```python
from build123d import *

# Parameters (mm, degrees)
SKETCH1_W           = 13.5
SKETCH1_H           = 13.5
BOSS_EXTRUDE1_DEPTH = 5
SKETCH3_W           = 13.5
SKETCH3_H           = 13.5
BOSS_EXTRUDE2_DEPTH = 2
CHAMFER1_SIZE       = 2.5
FILLET2_R           = 0.5
FILLET1_R           = 0.5
CUT_EXTRUDE1_REACH  = 4
SKETCH4_R           = 2.9
CHAMFER2_SIZE       = 0.2


with BuildPart() as part:
    # Sketch1 → Boss-Extrude1 (new body)
    with BuildSketch(Plane(origin=(0, 0, 0), x_dir=(1, 0, 0), z_dir=(0, 1, 0))):
        Rectangle(SKETCH1_W, SKETCH1_H)
        Polygon((0, -5.715767665), (4.95, -2.857883832), (4.95, 2.857883832), (0, 5.715767665), (-4.95, 2.857883832), (-4.95, -2.857883832), align=None, mode=Mode.SUBTRACT)
    extrude(amount=BOSS_EXTRUDE1_DEPTH)

    # Sketch3 → Boss-Extrude2 (add)
    with BuildSketch(Plane(origin=(0, 5, 0), x_dir=(1, 0, 0), z_dir=(0, 1, 0))):
        Rectangle(SKETCH3_W, SKETCH3_H)
    extrude(amount=BOSS_EXTRUDE2_DEPTH)

    # Chamfer1
    chamfer1_edges = [part.edges().sort_by_distance(p)[0] for p in [
        (-6.75, 7, 0),
        (6.75, 7, 0),
    ]]
    chamfer(chamfer1_edges, length=CHAMFER1_SIZE)

    # Fillet2
    fillet2_edges = [part.edges().sort_by_distance(p)[0] for p in [
        (-4.95, 2.5, 2.857883832),
        (0, 2.5, 5.715767665),
        (4.95, 2.5, 2.857883832),
        (4.95, 2.5, -2.857883832),
        (0, 2.5, -5.715767665),
        (-4.95, 2.5, -2.857883832),
    ]]
    fillet(fillet2_edges, radius=FILLET2_R)

    # Fillet1
    fillet1_edges = [part.edges().sort_by_distance(p)[0] for p in [
        (0, 7, 6.75),
        (0, 7, -6.75),
        (-4.25, 7, 0),
        (4.25, 7, 0),
        (-6.75, 2.25, -6.75),
        (6.75, 2.25, -6.75),
        (-5.5, 5.75, -6.75),
        (5.5, 5.75, -6.75),
        (6.75, 2.25, 6.75),
        (6.75, 4.5, 0),
        (-6.75, 2.25, 6.75),
        (-5.5, 5.75, 6.75),
        (5.5, 5.75, 6.75),
        (-6.75, 4.5, 0),
    ]]
    fillet(fillet1_edges, radius=FILLET1_R)

    # Sketch4 → Cut-Extrude1 (cut, up to next)
    with BuildSketch(Plane.XZ.offset(-5), mode=Mode.PRIVATE) as cut_extrude1_sk1:
        Circle(SKETCH4_R)
    cut_extrude1_tool1 = extrude(cut_extrude1_sk1.sketch, amount=-CUT_EXTRUDE1_REACH, mode=Mode.PRIVATE) & part.part
    add(cut_extrude1_tool1.solids().sort_by_distance((0, 5, 0))[0], mode=Mode.SUBTRACT)

    # Chamfer2
    chamfer2_edges = [part.edges().sort_by_distance(p)[0] for p in [
        (-2.9, 5, 0),
    ]]
    chamfer(chamfer2_edges, length=CHAMFER2_SIZE)


solid = part.part
```
Could you check a few things on this model? Use its own coordinates, in mm. A direction names the side the tool comes from. Coordinates: 2 decimals unless noted, no trailing zeros. Write each loop counter-clockwise with the first axis right and the second up, starting at its lowest first coordinate (ties: lowest second). Pieces come first, ordered by that corner, then holes. Notation, with made-up numbers: (-16.75, 2.5) -> (32.25, 2.5) arc R21 ccw to (32.25, 40.5) -> close; hole circle Ø7 at (52, -1.5). An arc over 180 degrees is marked (long way). Return JSON: item names as keys, results as strings.
(1) Imagine slicing it at A-A, the plane x = 0. Please give me the cut outline in (y, z), then the cut area to 3 significant figures.
Numbers:
{"outline": "(0, -6.75) -> (6.5, -6.75) arc R0.5 ccw to (7, -6.25) -> (7, -2.9) -> (5.2, -2.9) -> (5, -3.1) -> (5, -5.64) -> (0, -5.64) -> close; (0, 5.64) -> (5, 5.64) -> (5, 3.1) -> (5.2, 2.9) -> (7, 2.9) -> (7, 6.25) arc R0.5 ccw to (6.5, 6.75) -> (0, 6.75) -> close", "area": "26.4 mm2"}
(2) Which directions (+Z, -Z, +X, -X, +Y, -Y) give clear straight access to the entire face, cutting with the end or side of a thin tool? Please do faces 4 (the cylindrical face through (5.378, 5.659, -6.607)), 5 (the flat face through (-2.506, 2.465, 4.269)).
Numbers:
{"face 4": "-Z, +X, +Y", "face 5": "-Y"}
(3) We'd pull the mould along Z, two halves only. Please class faces 1 (the flat face through (6.75, 2, 0)), 2 (the flat face through (2.444, 2.465, 4.305)), 3 (the flat face through (0, 3, -6.75)): +Z half, -Z half, draft (parallel to the pull), parting line (faces both ways), or undercut.
Numbers:
{"face 1": "draft", "face 2": "undercut", "face 3": "-Z half"}
(4) I'm going to push a flat-ended pin straight in: pin 1 (6.5 mm diameter, centred on x = 0, z = 0, fed in from -Y). Where does the tip first touch, or does it pass through?
Numbers:
{"pin 1": "stops at y = 5"}
(5) I need wall thicknesses on L1, parallel to X at y = 3, z = 2; L2, parallel to Z at x = 0, y = 5.75; L3, parallel to X at y = 1.25, z = -4.75. Which ranges of each line are inside material? Lowest first, please.
Numbers:
{"L1": "x = -6.75 to -4.95, 4.95 to 6.75", "L2": "z = -6.75 to -2.9, 2.9 to 6.75", "L3": "x = -6.75 to -1.67, 1.67 to 6.75"}
(6) Imagine slicing it at C-C, the plane y = 4. Please give me the cut outline in (x, z).
Numbers:
{"outline": "(-6.75, -6.25) arc R0.5 ccw to (-6.25, -6.75) -> (6.25, -6.75) arc R0.5 ccw to (6.75, -6.25) -> (6.75, 6.25) arc R0.5 ccw to (6.25, 6.75) -> (-6.25, 6.75) arc R0.5 ccw to (-6.75, 6.25) -> close; hole (-4.95, -2.57) arc R0.5 ccw to (-4.7, -3) -> (-0.25, -5.57) arc R0.5 ccw to (0.25, -5.57) -> (4.7, -3) arc R0.5 ccw to (4.95, -2.57) -> (4.95, 2.57) arc R0.5 ccw to (4.7, 3) -> (0.25, 5.57) arc R0.5 ccw to (-0.25, 5.57) -> (-4.7, 3) arc R0.5 ccw to (-4.95, 2.57) -> close"}
(7) Imagine slicing it at B-B, the plane z = 0. Please give me the cut outline in (x, y).
Numbers:
{"outline": "(-6.75, 0) -> (-4.95, 0) -> (-4.95, 5) -> (-3.1, 5) -> (-2.9, 5.2) -> (-2.9, 7) -> (-4.04, 7) arc R0.5 ccw to (-4.4, 6.85) -> (-6.6, 4.65) arc R0.5 ccw to (-6.75, 4.29) -> close; (2.9, 5.2) -> (3.1, 5) -> (4.95, 5) -> (4.95, 0) -> (6.75, 0) -> (6.75, 4.29) arc R0.5 ccw to (6.6, 4.65) -> (4.4, 6.85) arc R0.5 ccw to (4.04, 7) -> (2.9, 7) -> close"}
(8) Imagine slicing it at D-D, the plane z = 3.5. Please give me the cut outline in (x, y), then the cut area to 3 significant figures.
Numbers:
{"outline": "(-6.75, 0) -> (-3.84, 0) -> (-3.84, 5) -> (3.84, 5) -> (3.84, 0) -> (6.75, 0) -> (6.75, 4.29) arc R0.5 ccw to (6.6, 4.65) -> (4.4, 6.85) arc R0.5 ccw to (4.04, 7) -> (-4.04, 7) arc R0.5 ccw to (-4.4, 6.85) -> (-6.6, 4.65) arc R0.5 ccw to (-6.75, 4.29) -> close", "area": "49.9 mm2"}
